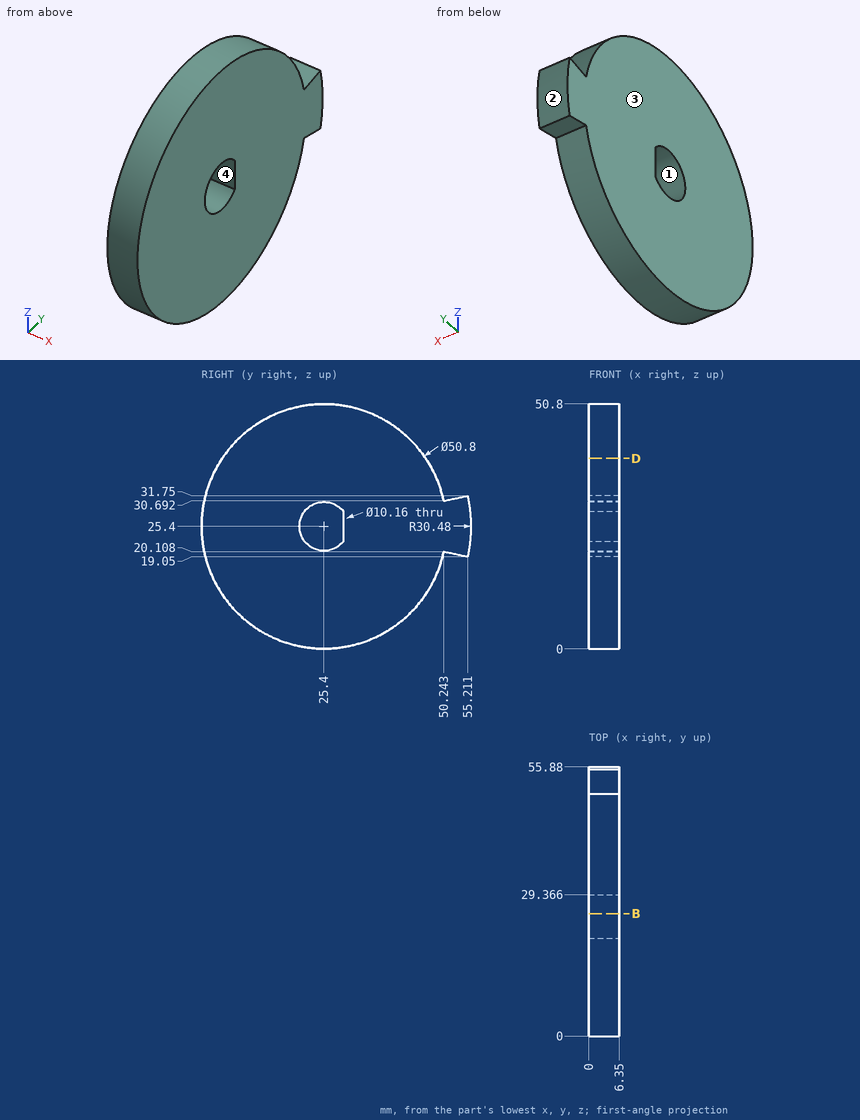
Geometry check sheet. Reference: drawing and pictorial views, mm from the part's lowest x, y, z. Round coordinates to 2 decimals unless told otherwise and drop trailing zeros. Write each loop counter-clockwise with the first axis right and the second up, starting at its lowest first coordinate (ties: lowest second). Pieces come first, ordered by that corner, then holes.
(1) Section check B-B (y = 25.4). Enter the section's corners in (x, z).
Returned:
outline: (0, 0) - (6.35, 0) - (6.35, 20.32) - (0, 20.32) - close; (0, 30.48) - (6.35, 30.48) - (6.35, 50.8) - (0, 50.8) - close
(2) Depth check by flat-ended pin: pin 1 Ø3 at (x, z) = (2, 26) entering from -Y; pin 2 Ø1.5 at (x, z) = (5.5, 22.5) entering from +Y; pin 3 Ø3 at (x, z) = (4.5, 39.5) entering from -Y (1 decimal). Enter the tip coordinate at first touch or a pass-through.
Returned:
pin 1: stops at y = 0
pin 2: stops at y = 55.8
pin 3: stops at y = 3.3
(3) Material ranges on line 1 (Z direction, x = 2, y = 25.4); line 2 (Y direction, x = 3, z = 25.4) (1 decimal); line 3 (Z direction, x = 3.75, y = 23) (1 decimal), recorded low to high.
Returned:
line 1: z = 0 to 20.32, 30.48 to 50.8
line 2: y = 0 to 20.3, 29.4 to 55.9
line 3: z = 0.1 to 20.9, 29.9 to 50.7
(4) Section check D-D (z = 39.5). Enter the section's corners in (x, y).
Returned:
outline: (0, 4.27) - (6.35, 4.27) - (6.35, 46.53) - (0, 46.53) - close
(5) Mould release check, pull along Y, two halves, no side actions. Record for the marked faces 1, 2, 3 and 4: pulls with the +Y half, pulls with the -Y half, needs draft (parallel to the pull), parting line crosses it, or undercut.
Returned:
face 1: undercut
face 2: pulls with the +Y half
face 3: needs draft
face 4: undercut
